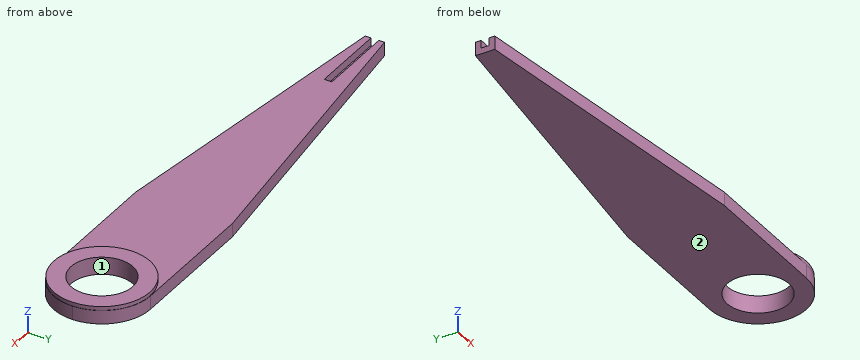
```python
from build123d import *

# Parameters (mm, degrees)
F0_R     = 8
F1_DEPTH = 3.5
F2_R     = 12.430903
F2_R_2   = 8
F3_DEPTH = 1
F4_W     = 20
F4_H     = 2
F5_DEPTH = 2


with BuildPart() as f1:
    # F0 (on Top) → F1 (new body)
    with BuildSketch(Plane.XY):
        with BuildLine():
            ThreePointArc((0, -12.5), (8.838835, -8.838835), (12.5, 0))
            ThreePointArc((12.5, 0), (8.838835, 8.838835), (0, 12.5))
            ThreePointArc((0, 12.5), (-12.5, 0), (0, -12.5))
        make_face()
        Circle(F0_R, mode=Mode.SUBTRACT)
        with BuildLine():
            ThreePointArc((0, -12.5), (-12.5, 0), (0, 12.5))
            Line((0, 12.5), (-35, 12.5))
            Line((-35, 12.5), (-116.388784, 2.506714))
            Line((-116.388784, 2.506714), (-116.388784, -2.506714))
            Line((-116.388784, -2.506714), (-35, -12.5))
            Line((-35, -12.5), (0, -12.5))
        make_face()
    extrude(amount=F1_DEPTH)

    # F2 (on face) → F3 (join)
    with BuildSketch(Plane.XY.offset(3.5)):
        Circle(F2_R)
        Circle(F2_R_2, mode=Mode.SUBTRACT)
    extrude(amount=F3_DEPTH)

    # F4 (on face) → F5 (cut)
    with BuildSketch(Plane.XY.offset(3.5)):
        with Locations((-106.388784, 0.006714)):
            Rectangle(F4_W, F4_H)
    extrude(amount=-F5_DEPTH, mode=Mode.SUBTRACT)


solid = f1.part
```
Could you check a few things on this model? Use its own coordinates, in mm. Face numbers are marked on the shaded views. Coordinates: 2 decimals unless noted, no trailing zeros. Loops run counter-clockwise (first coordinate to the right, second up) from the corner with the lowest first, then second, coordinate; pieces in that order, holes last. Notation, with made-up numbers: M -6,47.5 L 26,47.5 A19 cw 26,75.5 Z; hole C 24.25,37 d5. An arc over 180 degrees is marked long. Put each result on its own line as item: value. Start each with the question number.
(1) Thinking about a two-plate mould opening in X: for the marked faces 1 and 2, which applies, pulls with the +X half, pulls with the -X half, needs draft (parallel to the pull), parting line crosses it, or undercut?
(2) I need wall thicknesses on line 1 (Y direction, x = 0, z = 2.9); line 2 (Z direction, x = -61, y = 3.5); line 3 (Y direction, x = 0, z = 3.6). Which ranges of each line are inside material? Lowest first, please. Write a range as from..to.
(3) Suppose I cut it at B-B on y = -10. Please give me the cut outline in (x, z).
(4) Suppose I cut it at D-D on x = -50. Please give me the cut outline in (y, z).
(5) Suppose I cut it at C-C on x = -30. Please give me the cut outline in (y, z), then the cut area to 3 significant figures.
(6) Suppose I cut it at A-A on z = 0.75. Please give me the cut outline in (x, y), then the cut area to 3 significant figures.
(7) Will these pins go through, and if not, where does the flat tip stop? P1, Ø1.5, axis at x = -43, z = 3, coming from the -Y side; P2, Ø1, axis at x = -106, z = 2.5, coming from the +Y side; P3, Ø2, axis at x = -109, z = 2, coming from the -Y side.
Solutions:
1. face 1: undercut
1. face 2: needs draft
2. line 1: y = -12.5..-8, 8..12.5
2. line 2: z = 0..3.5
2. line 3: y = -12.43..-8, 8..12.43
3. outline: M -55.36,0 L 7.5,0 L 7.5,3.5 L 7.38,3.5 L 7.38,4.5 L -7.38,4.5 L -7.38,3.5 L -55.36,3.5 Z
4. outline: M -10.66,0 L 10.66,0 L 10.66,3.5 L -10.66,3.5 Z
5. outline: M -12.5,0 L 12.5,0 L 12.5,3.5 L -12.5,3.5 Z
5. area: 87.5 mm2
6. outline: M -116.39,-2.51 L -35,-12.5 L 0,-12.5 A12.5 ccw 12.5,0 A12.5 ccw 0,12.5 L -35,12.5 L -116.39,2.51 Z; hole C 0,0 d16
6. area: 2,140 mm2
7. P1: stops at y = -11.61
7. P2: stops at y = 3.84
7. P3: stops at y = -3.54
